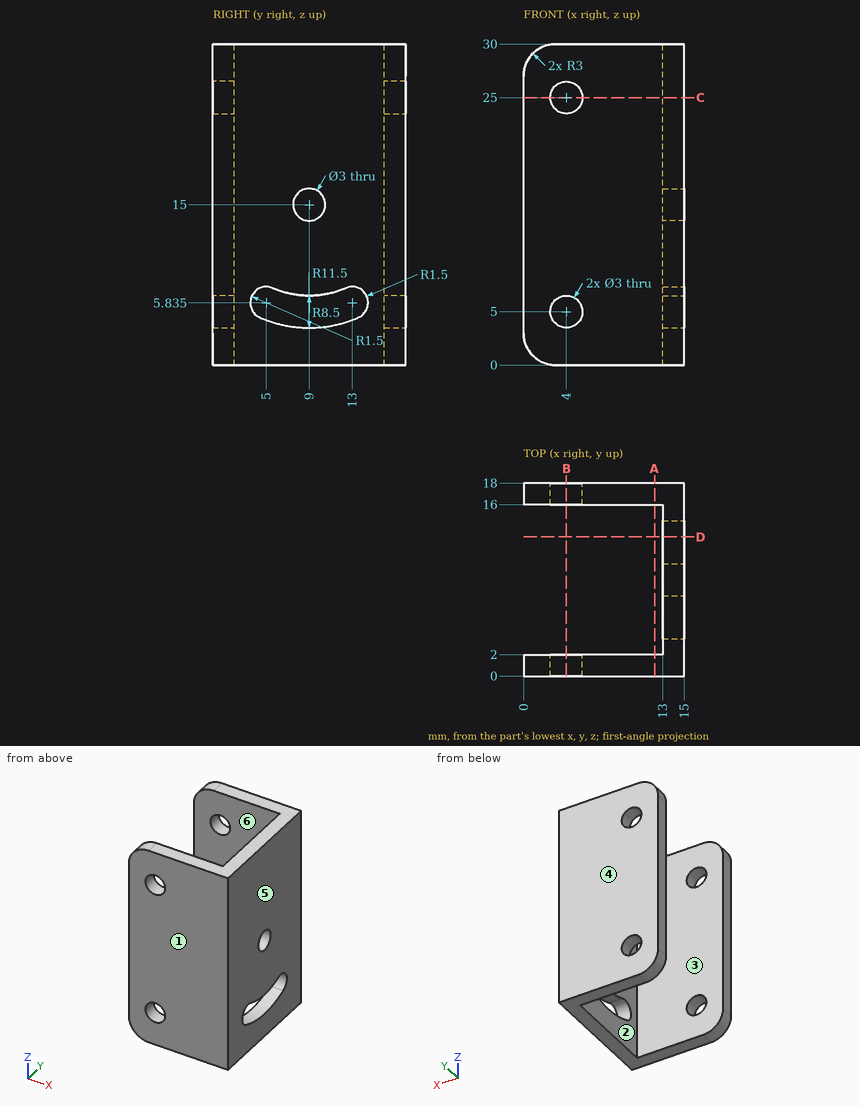
Here's the drawing with two shaded views (mm, measured from the low corner). I have some questions. A direction names the side the tool comes from. Give positions to 0.01 mm unless a question says otherwise; leave off trailing zeros. Order: outer loops, then holes, each group sorted by start corner. A loop starts at its lowest first (then second) coordinate and runs counter-clockwise, first axis right, second up.
Q1. Suppose I cut it at B-B, the plane x = 4. Write out the boundary of the cut face in (y, z), and give its area (3 significant figures).
Q2. Suppose I cut it at D-D, the plane y = 13. Write out the boundary of the cut face in (x, z) (3 decimals).
Q3. We'd pull the mould along Y, two halves only. Please class the marked faces 3, 4, 5 and 6: +Y half, -Y half, draft (parallel to the pull), parting line (faces both ways), or undercut.
Q4. I'm going to push a flat-ended pin straight in: P1, Ø4, axis at y = 10, z = 9, coming from the -X side. Where does the tip first touch, or does it pass through?
Q5. If I drill on line 1 along Y through (x, z) = (6.25, 15); line 2 along Y through (x, z) = (14.1, 15); line 3 along X through (y, z) = (5.5, 23.25), over which ranges is the centre line in solid material (lowest first)?
Q6. Suppose I cut it at A-A, the plane x = 12.25. Write out the boundary of the cut face in (y, z).
Q7. For the marked faces 1 and 2, which set-ups out of +Z, -Z, +X, -X, +Y, -Y let a thin tool reach every point of the face, with its end or its side?
Q8. Suppose I cut it at C-C, the plane z = 25. Write out the boundary of the cut face in (x, y), and give its area (3 significant figures).
Solution:
1. outline: (0, 0) - (2, 0) - (2, 3.5) - (0, 3.5) - close; (0, 6.5) - (2, 6.5) - (2, 23.5) - (0, 23.5) - close; (0, 26.5) - (2, 26.5) - (2, 30) - (0, 30) - close; (16, 0) - (18, 0) - (18, 3.5) - (16, 3.5) - close; (16, 6.5) - (18, 6.5) - (18, 23.5) - (16, 23.5) - close; (16, 26.5) - (18, 26.5) - (18, 30) - (16, 30) - close
1. area: 96.0 mm2
2. outline: (13, 0) - (15, 0) - (15, 4.218) - (13, 4.218) - close; (13, 7.335) - (15, 7.335) - (15, 30) - (13, 30) - close
3. face 3: undercut
3. face 4: +Y half
3. face 5: draft
3. face 6: undercut
4. P1: stops at x = 13
5. line 1: y = 0 to 2, 16 to 18
5. line 2: y = 0 to 7.5, 10.5 to 18
5. line 3: x = 13 to 15
6. outline: (0, 0) - (2, 0) - (2, 30) - (0, 30) - close; (16, 0) - (18, 0) - (18, 30) - (16, 30) - close
7. face 1: +Z, -Z, +X, -X, -Y
7. face 2: +Z, -Z, -X
8. outline: (0, 0) - (2.5, 0) - (2.5, 2) - (0, 2) - close; (0, 16) - (2.5, 16) - (2.5, 18) - (0, 18) - close; (5.5, 0) - (15, 0) - (15, 18) - (5.5, 18) - (5.5, 16) - (13, 16) - (13, 2) - (5.5, 2) - close
8. area: 76.0 mm2
